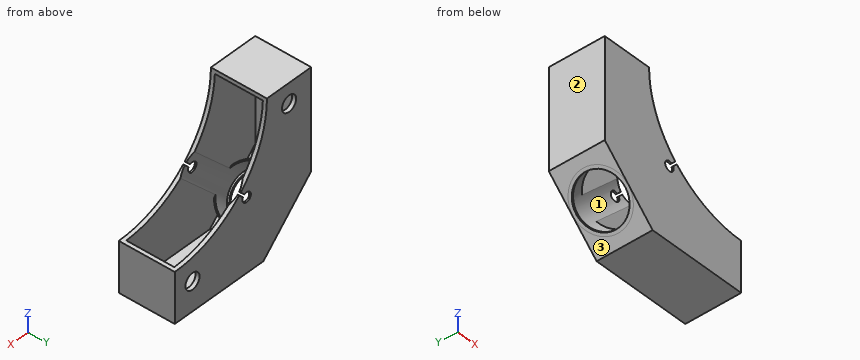
from build123d import *

# Parameters (mm, degrees)
BOSS_EXTRUDE1_DEPTH      = 28
SHELL1_T                 = -2
CUT_EXTRUDE1_DEPTH       = 12
CUT_EXTRUDE1_DEPTH_BACK  = 12
SKETCH9_R                = 6.4
SKETCH12_R               = 4
CUT_EXTRUDE3_DEPTH       = 2
BOSS_EXTRUDE2_DEPTH      = 0.0001
BOSS_EXTRUDE2_DEPTH_BACK = 10
SKETCH11_R               = 13.85
CUT_EXTRUDE4_DEPTH       = 35
CUT_EXTRUDE4_DEPTH_BACK  = 9
SKETCH13_R               = 13.25
CUT_EXTRUDE5_DEPTH       = 10
CUT_EXTRUDE5_DEPTH_BACK  = 10
SKETCH15_R               = 12.25


with BuildPart() as part:
    # Sketch1 → Boss-Extrude1 (new body)
    with BuildSketch(Plane(origin=(0, 0, 0), x_dir=(1, 0, 0), z_dir=(0, 1, 0))):
        with BuildLine():
            Line((0, 0), (0, 50))
            Line((0, 50), (27, 77))
            Line((27, 77), (77, 77))
            Line((77, 77), (77, 52))
            ThreePointArc((77, 52), (57.377961172, 48.155743087), (40.657159206, 37.191368932))
            Line((40.657159206, 37.191368932), (38.535838862, 39.312689275))
            ThreePointArc((38.535838862, 39.312689275), (34.771350846, 42.228649154), (37.687310725, 38.464161138))
            Line((37.687310725, 38.464161138), (39.808631068, 36.342840794))
            ThreePointArc((39.808631068, 36.342840794), (28.844256913, 19.622038828), (25, 0))
            Line((25, 0), (0, 0))
        make_face()
    extrude(amount=BOSS_EXTRUDE1_DEPTH)

    # Shell1
    shell1_openings = [part.faces().sort_by_distance(p)[0] for p in [
        (57.377961172, 14, -48.155743087),
        (28.844256913, 14, -19.622038828),
    ]]
    offset(amount=SHELL1_T, openings=shell1_openings, kind=Kind.INTERSECTION)

    # Sketch9 → Cut-Extrude1 (cut, two sides: drawn at the far end of the back side and taken through both)
    with BuildSketch(Plane(origin=(0, 14, 0), x_dir=(1, 0, 0), z_dir=(0, 1, 0)).offset(-CUT_EXTRUDE1_DEPTH_BACK)):
        with Locations((36.184678266, 38.815321734)):
            Circle(SKETCH9_R)
    extrude(amount=CUT_EXTRUDE1_DEPTH + CUT_EXTRUDE1_DEPTH_BACK, mode=Mode.SUBTRACT)

    # Sketch12 → Cut-Extrude3 (cut)
    with BuildSketch(Plane(origin=(0, 28, 0), x_dir=(1, 0, 0), z_dir=(0, 1, 0))):
        with Locations(Location((67, 62.5, 0), (0, 0, 270))):
            Circle(SKETCH12_R)
        with Locations(Location((12.5, 10, 0), (0, 0, 270))):
            Circle(SKETCH12_R)
    extrude(amount=-CUT_EXTRUDE3_DEPTH, mode=Mode.SUBTRACT)

    # Sketch11 → Boss-Extrude2 (add, two sides: drawn at the far end of the back side and taken through both)
    with BuildSketch(Plane(origin=(-25, 0, -25), x_dir=(-0.7071067811865435, 0, 0.7071067811865517), z_dir=(-0.7071067811865517, 0, -0.7071067811865435)).offset(-BOSS_EXTRUDE2_DEPTH_BACK)):
        with Locations((-54.447222151, 14)):
            Circle(SKETCH11_R)
    extrude(amount=BOSS_EXTRUDE2_DEPTH + BOSS_EXTRUDE2_DEPTH_BACK)

    # Sketch13 → Cut-Extrude4 (cut, two sides: drawn at the far end of the back side and taken through both)
    with BuildSketch(Plane(origin=(-17.928932188, 0, -17.928932188), x_dir=(0.7071067811865435, 0, -0.7071067811865516), z_dir=(0.7071067811865516, 0, 0.7071067811865435)).offset(-CUT_EXTRUDE4_DEPTH_BACK)):
        with Locations(Location((54.447222151, 14, 0), (0, 0, 115.087627842))):
            Circle(SKETCH13_R)
    extrude(amount=CUT_EXTRUDE4_DEPTH + CUT_EXTRUDE4_DEPTH_BACK, mode=Mode.SUBTRACT)

    # Sketch15 → Cut-Extrude5 (cut, two sides: drawn at the far end of the back side and taken through both)
    with BuildSketch(Plane(origin=(-25, 0, -25), x_dir=(-0.7071067811865435, 0, 0.7071067811865517), z_dir=(-0.7071067811865517, 0, -0.7071067811865435)).offset(-CUT_EXTRUDE5_DEPTH_BACK)):
        with Locations(Location((-54.447222151, 14, 0), (0, 0, 180))):
            Circle(SKETCH15_R)
    extrude(amount=CUT_EXTRUDE5_DEPTH + CUT_EXTRUDE5_DEPTH_BACK, mode=Mode.SUBTRACT)


solid = part.part
Could you check a few things on this model? Use its own coordinates, in mm. Face numbers are marked on the shaded views. Round coordinates to 2 decimals unless told otherwise and drop trailing zeros. Order: outer loops, then holes, each group sorted by start corner. A loop starts at its lowest first (then second) coordinate and runs counter-clockwise, first axis right, second up.
(1) If we mould it in two halves opening along Z, with no side actions, what happens to the marked faces 1, 2 and 3? For each: released by +Z, released by -Z, zero draft, split by the parting line, or undercut.
Response values:
face 1: undercut
face 2: zero draft
face 3: released by -Z
(2) I'm going to push flat-ended pins straight in: pin 1 (10.5 mm diameter, centred on x = 57, z = -64, fed in from -Y); pin 2 (6 mm diameter, centred on x = 59, y = 16, fed in from +Z); pin 3 (7 mm diameter, centred on y = 10, z = -61, fed in from -X); pin 4 (7 mm diameter, centred on x = 10.5, y = 15.5, fed in from -Z). Where does each tip first touch, or does it pass through?
Response values:
pin 1: stops at y = 0
pin 2: stops at z = -75
pin 3: stops at x = 75
pin 4: stops at z = -51.45
(3) Imagine slicing it at A-A (z = -7). Write out the boundary of the cut face in (x, y), plus the area to 3 significant figures.
Response values:
outline: (0, 0) - (25.47, 0) - (25.47, 2) - (2, 2) - (2, 26) - (9.85, 26) - (9.85, 28) - (0, 28) - close; (15.15, 26) - (25.47, 26) - (25.47, 28) - (15.15, 28) - close
area: 139 mm2
(4) Imagine slicing it at D-D (z = -28.5). Write out the boundary of the cut face in (x, y), plus the area to 3 significant figures.
Response values:
outline: (0, 0) - (33.51, 0) - (33.51, 2) - (2, 2) - (2, 26) - (33.51, 26) - (33.51, 28) - (0, 28) - close
area: 182 mm2
(5) Please list where these lines run through material, in increasing order: line 1 along Y through (x, z) = (61, -68); line 2 along Y through (x, z) = (19, -57); line 3 along Z through (x, y) = (24, 21.75).
Response values:
line 1: y = 0 to 2, 26 to 28
line 2: y = 0 to 0.77, 27.23 to 28
line 3: z = -74 to -71.17, -69.23 to -68.2, -2 to 0
(6) Imagine slicing it at C-C (x = 68). Write out the boundary of the cut face in (y, z).
Response values:
outline: (0, -77) - (28, -77) - (28, -66.37) - (26, -66.37) - (26, -75) - (2, -75) - (2, -51.22) - (0, -51.22) - close; (26, -58.63) - (28, -58.63) - (28, -51.22) - (26, -51.22) - close
